from build123d import *

# Parameters (mm, degrees)
BOSS_EXTRUDE1_DEPTH      = 7
SKETCH2_R                = 1.75
CUT_EXTRUDE1_DEPTH       = 25.760906688
CHAMFER1_SIZE            = 0.5
CHAMFER1_OF_MIRROR1_SIZE = 0.5
CUT_EXTRUDE2_DEPTH       = 26.304199256


with BuildPart() as part:
    # Sketch1 → Boss-Extrude1 (new body)
    with BuildSketch(Plane.XY):
        Polygon((0, 11.5), (11.55, 11.5), (11.55, 0), (21.05, 0), (21.05, 2), (13.05, 2), (13.05, 13), (0, 13), align=None)
    boss_extrude1 = extrude(amount=BOSS_EXTRUDE1_DEPTH)

    # Sketch2 → Cut-Extrude1 (cut, through all)
    with BuildSketch(Plane(origin=(0, 2, 0), x_dir=(1, 0, 0), z_dir=(0, 1, 0))):
        with Locations(Location((17.05, -3.5, 0), (0, 0, 180))):
            Circle(SKETCH2_R)
        with BuildLine():
            Line((17.05, 0), (21.05, 0))
            Line((21.05, 0), (21.05, -7))
            Line((21.05, -7), (17.05, -7))
            ThreePointArc((17.05, -7), (20.55, -3.5), (17.05, 0))
        make_face()
    cut_extrude1 = extrude(amount=-CUT_EXTRUDE1_DEPTH, mode=Mode.SUBTRACT)

    # Chamfer1
    chamfer1_edges = [part.edges().sort_by_distance(p)[0] for p in [
        (11.55, 0, 3.5),
        (13.05, 13, 3.5),
    ]]
    chamfer(chamfer1_edges, length=CHAMFER1_SIZE)

    # Mirror1: Boss-Extrude1, Cut-Extrude1 across plane
    add(boss_extrude1.mirror(Plane(origin=(0, 0, 0), x_dir=(0, 0, 1), z_dir=(1, 0, 0))))
    add(cut_extrude1.mirror(Plane(origin=(0, 0, 0), x_dir=(0, 0, 1), z_dir=(1, 0, 0))), mode=Mode.SUBTRACT)

    # Chamfer1 of Mirror1
    chamfer1_of_mirror1_edges = [part.edges().sort_by_distance(p)[0] for p in [
        (-11.55, 0, 3.5),
        (-13.05, 13, 3.5),
    ]]
    chamfer(chamfer1_of_mirror1_edges, length=CHAMFER1_OF_MIRROR1_SIZE)

    # Sketch3 → Cut-Extrude2 (cut, through all)
    with BuildSketch(Plane(origin=(0, 13, 0), x_dir=(1, 0, 0), z_dir=(0, 1, 0))):
        with BuildLine():
            Line((-2.5, 0), (2.5, 0))
            ThreePointArc((2.5, 0), (0, -2.5), (-2.5, 0))
        make_face()
    extrude(amount=-CUT_EXTRUDE2_DEPTH, mode=Mode.SUBTRACT)


solid = part.part
Input: part model. Units: mm. Frame: model coordinates. A direction names the side the tool comes from. Give positions to 0.01 mm unless a question says otherwise; leave off trailing zeros. Loops run counter-clockwise (first coordinate to the right, second up) from the corner with the lowest first, then second, coordinate; pieces in that order, holes last. Notation, with made-up numbers: (-2, 18) -> (34, 18) arc R29 cw to (34, 43) -> close; hole circle Ø4 at (86, 83.25). An arc over 180 degrees is marked (long way). Answer as a JSON object with one key per item and string values. Group by question number.
Item 1: Cut plane C-C, the plane z = 5.75. Return the cut outline in (x, y), and give its area (3 significant figures).
Item 2: Pull-direction query (X, two-part tool) for faces 4 (the flat face through (-12, 7, 0)), 5 (the cylindrical face through (-15.433, 1.014, 2.83)), 6 (the cylindrical face through (-20.55, 1.01, 3.58)), 7 (the cylindrical face through (20.55, 1.01, 3.58)); classes: released by +X, released by -X, zero draft, split by the parting line, or undercut.
Item 3: Reachability of faces 1 (the flat face through (15, 2, 3)), 2 (the flat face through (0, 11.5, 3)), 3 (the flat face through (-15, 2, 3)) from +Z, -Z, +X, -X, +Y, -Y: full face, straight path, thin tool, end or side. Return the list, or none.
Item 4: Cut plane B-B, the plane z = 3.5. Return the cut outline in (x, y), and give its area (4 significant figures).
Item 5: Cut plane D-D, the plane x = 0. Return the cut outline in (y, z), and give its area (3 significant figures).
Item 6: Cut plane A-A, the plane y = 3.5. Return the cut outline in (x, z), and give its area (3 significant figures).
Item 7: Pin query (flat end, axial travel): P1, Ø3.5, axis at y = 5.5, z = 5, coming from the -X side; P2, Ø1.5, axis at y = 11, z = 3, coming from the +X side; P3, Ø3.5, axis at x = -2, z = 3, coming from the -Y side. Return the tip coordinate at first contact, or that it passes through.
Item 8: Line query: probe 1 along Z at (x, y) = (17.05, 0.85); probe 2 along X at (y, z) = (9, 1.5); probe 3 along X at (y, z) = (1.5, 2.5). Output: solid intervals per line, ascending.
Checks:
{
 "1": {"outline": "(-19.73, 0) -> (-12.05, 0) -> (-11.55, 0.5) -> (-11.55, 11.5) -> (11.55, 11.5) -> (11.55, 0.5) -> (12.05, 0) -> (19.73, 0) -> (19.73, 2) -> (13.05, 2) -> (13.05, 12.5) -> (12.55, 13) -> (-12.55, 13) -> (-13.05, 12.5) -> (-13.05, 2) -> (-19.73, 2) -> close", "area": "99.9 mm²"},
 "2": {"face 4": "zero draft", "face 5": "undercut", "face 6": "released by -X", "face 7": "released by +X"},
 "3": {"face 1": "+Z, -Z, +X, +Y", "face 2": "+Z, -Z, -Y", "face 3": "+Z, -Z, -X, +Y"},
 "4": {"outline": "(-20.55, 0) -> (-18.8, 0) -> (-18.8, 2) -> (-20.55, 2) -> close; (-15.3, 0) -> (-12.05, 0) -> (-11.55, 0.5) -> (-11.55, 11.5) -> (11.55, 11.5) -> (11.55, 0.5) -> (12.05, 0) -> (15.3, 0) -> (15.3, 2) -> (13.05, 2) -> (13.05, 12.5) -> (12.55, 13) -> (-12.55, 13) -> (-13.05, 12.5) -> (-13.05, 2) -> (-15.3, 2) -> close; (18.8, 0) -> (20.55, 0) -> (20.55, 2) -> (18.8, 2) -> close", "area": "89.15 mm²"},
 "5": {"outline": "(11.5, 2.5) -> (13, 2.5) -> (13, 7) -> (11.5, 7) -> close", "area": "6.75 mm²"},
 "6": {"outline": "(-13.05, 0) -> (-11.55, 0) -> (-11.55, 7) -> (-13.05, 7) -> close; (11.55, 0) -> (13.05, 0) -> (13.05, 7) -> (11.55, 7) -> close", "area": "21.0 mm²"},
 "7": {"P1": "stops at x = -13.05", "P2": "stops at x = 13.05", "P3": "stops at y = 11.5"},
 "8": {"probe 1": "z = 0 to 1.75, 5.25 to 7", "probe 2": "x = -13.05 to -11.55, 11.55 to 13.05", "probe 3": "x = -20.4 to -18.49, -15.61 to -11.55, 11.55 to 15.61, 18.49 to 20.4"}
}
